from build123d import *

# Parameters (mm, degrees)
F0_R     = 8
F1_DEPTH = 5


with BuildPart() as f1:
    # F0 (on Top) → F1 (new body)
    with BuildSketch(Plane.XY):
        with BuildLine():
            ThreePointArc((-8.0044057119, 10.2435096134), (-6.5, 11.2583302492), (-4.8689366932, 12.0537734954))
            Line((-4.8689366932, 12.0537734954), (-4.7373265178, 12.1297586656))
            Line((-4.7373265178, 12.1297586656), (-6.4657635443, 14.018596429))
            Line((-6.4657635443, 14.018596429), (-8.933935945, 12.593596429))
            Line((-8.933935945, 12.593596429), (-8.0715243224, 10.2047586656))
            Line((-8.0715243224, 10.2047586656), (-8.0044057119, 10.2435096134))
        make_face()
        with BuildLine():
            ThreePointArc((4.743830128, 12.1035563252), (3.3556109574, 12.5594536148), (1.925, 12.8566860038))
            Line((1.925, 12.8566860038), (-1.925, 12.8566860038))
            ThreePointArc((-1.925, 12.8566860038), (-3.4206082897, 12.5419073082), (-4.8689366932, 12.0537734954))
            Line((-4.8689366932, 12.0537734954), (-8.0044057119, 10.2435096134))
            ThreePointArc((-8.0044057119, 10.2435096134), (-9.18182436, 9.2029398249), (-10.2250960025, 8.0279145325))
            Line((-10.2250960025, 8.0279145325), (-12.0649259258, 4.841235628))
            ThreePointArc((-12.0649259258, 4.841235628), (-12.5358348008, 3.4427962251), (-12.8452325787, 2))
            Line((-12.8452325787, 2), (-12.8452325787, -1.8141498167))
            Line((-12.8452325787, -1.8141498167), (-12.8735077012, -1.8090880212))
            ThreePointArc((-12.8735077012, -1.8090880212), (-12.5874883323, -3.2488671079), (-12.1409769307, -4.6472227372))
            Line((-12.1409769307, -4.6472227372), (-12.1183052404, -4.6264763345))
            Line((-12.1183052404, -4.6264763345), (-10.1933052404, -7.9606741391))
            Line((-10.1933052404, -7.9606741391), (-10.2590920013, -7.9844242941))
            ThreePointArc((-10.2590920013, -7.9844242941), (-9.280273641, -9.1036542744), (-8.1800560603, -10.1037954675))
            Line((-8.1800560603, -10.1037954675), (-8.15760444, -10.0327566781))
            Line((-8.15760444, -10.0327566781), (-4.8234066354, -11.9577566781))
            Line((-4.8234066354, -11.9577566781), (-4.8953676956, -12.0430633613))
            ThreePointArc((-4.8953676956, -12.0430633613), (-3.470885444, -12.5280866151), (-1.9998974916, -12.8452485388))
            Line((-1.9998974916, -12.8452485388), (-2.0243967581, -12.7343823954))
            Line((-2.0243967581, -12.7343823954), (1.8256032419, -12.7343823954))
            Line((1.8256032419, -12.7343823954), (1.8004811118, -12.874714279))
            ThreePointArc((1.8004811118, -12.874714279), (3.2879257328, -12.5773425005), (4.730605508, -12.1087312105))
            Line((4.730605508, -12.1087312105), (4.6379297596, -12.0074550572))
            Line((4.6379297596, -12.0074550572), (7.9721275642, -10.0824550572))
            Line((7.9721275642, -10.0824550572), (8.0245708298, -10.2277203226))
            ThreePointArc((8.0245708298, -10.2277203226), (9.1634355916, -9.2212498154), (10.1770488861, -8.0887376006))
            Line((10.1770488861, -8.0887376006), (10.0442101032, -8.0467542567))
            Line((10.0442101032, -8.0467542567), (11.9692101032, -4.7125564521))
            Line((11.9692101032, -4.7125564521), (12.0792509027, -4.8053821522))
            ThreePointArc((12.0792509027, -4.8053821522), (12.555754306, -3.3694263322), (12.8621959896, -1.8878332353))
            Line((12.8621959896, -1.8878332353), (12.7458358205, -1.9135465749))
            Line((12.7458358205, -1.9135465749), (12.7458358205, 1.9364534251))
            Line((12.7458358205, 1.9364534251), (12.8579739202, 1.9163785295))
            ThreePointArc((12.8579739202, 1.9163785295), (12.5521491468, 3.3828319198), (12.0796545351, 4.8043674205))
            Line((12.0796545351, 4.8043674205), (12.0189084823, 4.7487799429))
            Line((12.0189084823, 4.7487799429), (10.0939084823, 8.0829777475))
            Line((10.0939084823, 8.0829777475), (10.1620468907, 8.1075768878))
            ThreePointArc((10.1620468907, 8.1075768878), (9.1753494128, 9.2093953739), (8.0698840464, 10.1920052727))
            Line((8.0698840464, 10.1920052727), (8.0582076818, 10.1550602865))
            Line((8.0582076818, 10.1550602865), (4.7240098772, 12.0800602865))
            Line((4.7240098772, 12.0800602865), (4.743830128, 12.1035563252))
        make_face()
        Circle(F0_R, mode=Mode.SUBTRACT)
        with BuildLine():
            ThreePointArc((-12.0649259258, 4.841235628), (-11.2583302492, 6.5), (-10.2250960025, 8.0279145325))
            Line((-10.2250960025, 8.0279145325), (-10.1436068614, 8.1690578651))
            Line((-10.1436068614, 8.1690578651), (-12.5848961169, 8.9406208386))
            Line((-12.5848961169, 8.9406208386), (-14.0098961169, 6.4724484378))
            Line((-14.0098961169, 6.4724484378), (-12.0686068614, 4.8348600605))
            Line((-12.0686068614, 4.8348600605), (-12.0649259258, 4.841235628))
        make_face()
        with BuildLine():
            ThreePointArc((-12.8735077012, -1.8090880212), (-12.9996418521, 0.096497236), (-12.8452325787, 2))
            Line((-12.8452325787, 2), (-12.8452325787, 2.0358501833))
            Line((-12.8452325787, 2.0358501833), (-15.3452325787, 1.4833986912))
            Line((-15.3452325787, 1.4833986912), (-15.3452325787, -1.3666013088))
            Line((-15.3452325787, -1.3666013088), (-12.8735077012, -1.8090880212))
        make_face()
        with BuildLine():
            ThreePointArc((-10.2590920013, -7.9844242941), (-11.3236478485, -6.3855304715), (-12.1409769307, -4.6472227372))
            Line((-12.1409769307, -4.6472227372), (-14.0071430039, -6.354913361))
            Line((-14.0071430039, -6.354913361), (-12.5821430039, -8.8230857618))
            Line((-12.5821430039, -8.8230857618), (-10.2590920013, -7.9844242941))
        make_face()
        with BuildLine():
            ThreePointArc((-4.8953676956, -12.0430633613), (-6.6092258692, -11.1945582052), (-8.1800560603, -10.1037954675))
            Line((-8.1800560603, -10.1037954675), (-8.9291674135, -12.4740459336))
            Line((-8.9291674135, -12.4740459336), (-6.4609950127, -13.8990459336))
            Line((-6.4609950127, -13.8990459336), (-4.8953676956, -12.0430633613))
        make_face()
        with BuildLine():
            ThreePointArc((1.8004811118, -12.874714279), (-0.1007907763, -12.9996092718), (-1.9998974916, -12.8452485388))
            Line((-1.9998974916, -12.8452485388), (-1.4719452661, -15.2343823954))
            Line((-1.4719452661, -15.2343823954), (1.3780547339, -15.2343823954))
            Line((1.3780547339, -15.2343823954), (1.8004811118, -12.874714279))
        make_face()
        with BuildLine():
            Line((8.8345391869, -12.4712928206), (8.0245708298, -10.2277203226))
            ThreePointArc((8.0245708298, -10.2277203226), (6.4465635297, -11.2890131835), (4.730605508, -12.1087312105))
            Line((4.730605508, -12.1087312105), (6.3663667861, -13.8962928206))
            Line((6.3663667861, -13.8962928206), (8.8345391869, -12.4712928206))
        make_face()
        with BuildLine():
            Line((13.9104993587, -6.3501448294), (12.0792509027, -4.8053821522))
            ThreePointArc((12.0792509027, -4.8053821522), (11.2485921707, -6.5168377437), (10.1770488861, -8.0887376006))
            Line((10.1770488861, -8.0887376006), (12.4854993587, -8.8183172302))
            Line((12.4854993587, -8.8183172302), (13.9104993587, -6.3501448294))
        make_face()
        with BuildLine():
            Line((15.2458358205, 1.4889049172), (12.8579739202, 1.9163785295))
            ThreePointArc((12.8579739202, 1.9163785295), (12.9644448582, 0.96081711), (13, 0))
            ThreePointArc((13, 0), (12.9655032271, -0.9464280571), (12.8621959896, -1.8878332353))
            Line((12.8621959896, -1.8878332353), (15.2458358205, -1.3610950828))
            Line((15.2458358205, -1.3610950828), (15.2458358205, 1.4889049172))
        make_face()
        with BuildLine():
            Line((6.3615982545, 14.021349542), (4.743830128, 12.1035563252))
            ThreePointArc((4.743830128, 12.1035563252), (6.4777561387, 11.2711434827), (8.0698840464, 10.1920052727))
            Line((8.0698840464, 10.1920052727), (8.8297706553, 12.596349542))
            Line((8.8297706553, 12.596349542), (6.3615982545, 14.021349542))
        make_face()
        with BuildLine():
            ThreePointArc((-1.925, 12.8566860038), (0, 13), (1.925, 12.8566860038))
            Line((1.925, 12.8566860038), (1.3725485079, 15.3566860038))
            Line((1.3725485079, 15.3566860038), (-1.4774514921, 15.3566860038))
            Line((-1.4774514921, 15.3566860038), (-1.925, 12.8566860038))
        make_face()
        with BuildLine():
            Line((12.4827462457, 8.9453893702), (10.1620468907, 8.1075768878))
            ThreePointArc((10.1620468907, 8.1075768878), (11.2428252132, 6.5267818429), (12.0796545351, 4.8043674205))
            Line((12.0796545351, 4.8043674205), (13.9077462457, 6.4772169694))
            Line((13.9077462457, 6.4772169694), (12.4827462457, 8.9453893702))
        make_face()
        with BuildLine():
            ThreePointArc((13, 0), (12.9644448582, 0.96081711), (12.8579739202, 1.9163785295))
            Line((12.8579739202, 1.9163785295), (12.7458358205, 1.9364534251))
            Line((12.7458358205, 1.9364534251), (12.7458358205, -1.9135465749))
            Line((12.7458358205, -1.9135465749), (12.8621959896, -1.8878332353))
            ThreePointArc((12.8621959896, -1.8878332353), (12.9655032271, -0.9464280571), (13, 0))
        make_face()
        with BuildLine():
            ThreePointArc((12.0796545351, 4.8043674205), (11.2428252132, 6.5267818429), (10.1620468907, 8.1075768878))
            Line((10.1620468907, 8.1075768878), (10.0939084823, 8.0829777475))
            Line((10.0939084823, 8.0829777475), (12.0189084823, 4.7487799429))
            Line((12.0189084823, 4.7487799429), (12.0796545351, 4.8043674205))
        make_face()
        with BuildLine():
            ThreePointArc((8.0698840464, 10.1920052727), (6.4777561387, 11.2711434827), (4.743830128, 12.1035563252))
            Line((4.743830128, 12.1035563252), (4.7240098772, 12.0800602865))
            Line((4.7240098772, 12.0800602865), (8.0582076818, 10.1550602865))
            Line((8.0582076818, 10.1550602865), (8.0698840464, 10.1920052727))
        make_face()
        with BuildLine():
            Line((-1.925, 12.8566860038), (1.925, 12.8566860038))
            ThreePointArc((1.925, 12.8566860038), (0, 13), (-1.925, 12.8566860038))
        make_face()
        with BuildLine():
            Line((-8.0044057119, 10.2435096134), (-4.8689366932, 12.0537734954))
            ThreePointArc((-4.8689366932, 12.0537734954), (-6.5, 11.2583302492), (-8.0044057119, 10.2435096134))
        make_face()
        with BuildLine():
            Line((-12.0649259258, 4.841235628), (-10.2250960025, 8.0279145325))
            ThreePointArc((-10.2250960025, 8.0279145325), (-11.2583302492, 6.5), (-12.0649259258, 4.841235628))
        make_face()
        with BuildLine():
            Line((-12.8452325787, -1.8141498167), (-12.8452325787, 2))
            ThreePointArc((-12.8452325787, 2), (-12.9996418521, 0.096497236), (-12.8735077012, -1.8090880212))
            Line((-12.8735077012, -1.8090880212), (-12.8452325787, -1.8141498167))
        make_face()
        with BuildLine():
            Line((-12.1183052404, -4.6264763345), (-12.1409769307, -4.6472227372))
            ThreePointArc((-12.1409769307, -4.6472227372), (-11.3236478485, -6.3855304715), (-10.2590920013, -7.9844242941))
            Line((-10.2590920013, -7.9844242941), (-10.1933052404, -7.9606741391))
            Line((-10.1933052404, -7.9606741391), (-12.1183052404, -4.6264763345))
        make_face()
        with BuildLine():
            Line((-8.15760444, -10.0327566781), (-8.1800560603, -10.1037954675))
            ThreePointArc((-8.1800560603, -10.1037954675), (-6.6092258692, -11.1945582052), (-4.8953676956, -12.0430633613))
            Line((-4.8953676956, -12.0430633613), (-4.8234066354, -11.9577566781))
            Line((-4.8234066354, -11.9577566781), (-8.15760444, -10.0327566781))
        make_face()
        with BuildLine():
            Line((-2.0243967581, -12.7343823954), (-1.9998974916, -12.8452485388))
            ThreePointArc((-1.9998974916, -12.8452485388), (-0.1007907763, -12.9996092718), (1.8004811118, -12.874714279))
            Line((1.8004811118, -12.874714279), (1.8256032419, -12.7343823954))
            Line((1.8256032419, -12.7343823954), (-2.0243967581, -12.7343823954))
        make_face()
        with BuildLine():
            ThreePointArc((4.730605508, -12.1087312105), (6.4465635297, -11.2890131835), (8.0245708298, -10.2277203226))
            Line((8.0245708298, -10.2277203226), (7.9721275642, -10.0824550572))
            Line((7.9721275642, -10.0824550572), (4.6379297596, -12.0074550572))
            Line((4.6379297596, -12.0074550572), (4.730605508, -12.1087312105))
        make_face()
        with BuildLine():
            ThreePointArc((10.1770488861, -8.0887376006), (11.2485921707, -6.5168377437), (12.0792509027, -4.8053821522))
            Line((12.0792509027, -4.8053821522), (11.9692101032, -4.7125564521))
            Line((11.9692101032, -4.7125564521), (10.0442101032, -8.0467542567))
            Line((10.0442101032, -8.0467542567), (10.1770488861, -8.0887376006))
        make_face()
    extrude(amount=F1_DEPTH)


solid = f1.part
Geometry: final body of the model. Coordinates: model frame, mm. A direction names the side the tool comes from. Round coordinates to 2 decimals unless told otherwise and drop trailing zeros. Loops run counter-clockwise (first coordinate to the right, second up) from the corner with the lowest first, then second, coordinate; pieces in that order, holes last. Notation, with made-up numbers: M 27.25,27 L 64.25,27 A25 cw 64.25,50 Z; hole C -7,60.5 d2. An arc over 180 degrees is marked long. One line per question, with ' | ' between items.
(1) Cut plane B-B on x = 0. Return the cut outline in (y, z).
Check result:
outline: M -15.23,0 L -8,0 L -8,5 L -15.23,5 Z; M 8,0 L 15.36,0 L 15.36,5 L 8,5 Z
(2) Contact query for flat-ended pins moving along their axis: P1, Ø1.5, axis at y = -5, z = 4, coming from the -X side; P2, Ø9.5, axis at x = 0, y = 0, coming from the +Z side. Output: stop coordinate, or through.
Check result:
P1: stops at x = -13.35 | P2: passes through
(3) Cut plane A-A on y = 0. Return the cut outline in (x, z), plus the area to 3 significant figures.
Check result:
outline: M -15.35,0 L -8,0 L -8,5 L -15.35,5 Z; M 8,0 L 15.25,0 L 15.25,5 L 8,5 Z | area: 73.0 mm2
(4) Pull-direction query (X, two-part tool) for faces 1 (the flat face through (12.98, 5.63, 2.46)), 2 (the flat face through (5.564, 13.076, 2.465)), 3 (the flat face through (7, -7, 0)); classes: +X half, -X half, draft (parallel to the pull), parting line (faces both ways), or undercut.
Check result:
face 1: +X half | face 2: undercut | face 3: draft
(5) Material intervals for line 1 along Y through (x, z) = (0, 1.75); line 2 along X through (y, z) = (-13, 2.45); line 3 along Y through (x, z) = (-5, 0.95) (3 decimals), sorted ascending. Write a range as from..to.
Check result:
line 1: y = -15.23..-8, 8..15.36 | line 2: x = -8.02..-5.7, -1.97..1.78, 5.55..7.92 | line 3: y = -12.167..-6.245, 6.245..12.417
(6) Access query for faces 4 (the flat face through (8.445, 11.377, 2.465)), 5 (the flat face through (-14.127, -1.585, 2.465)), 6 (the cylindrical face through (-3.491, -12.522, 2.465)), 7 (the flat face through (7.61, 13.3, 2.46)). Directions: +Z, -Z, +X, -X, +Y, -Y. A direction counts if a zero-diameter tool reaches every point of the face in a straight line with its end or side. Return the directions, or none.
Check result:
face 4: +Z, -Z, +X | face 5: +Z, -Z, -X | face 6: +Z, -Z, -Y | face 7: +Z, -Z, +X, +Y
